The model under review builds one solid part; all positions refer to its coordinate system, in mm. A direction names the side the tool comes from. Give positions to 0.01 mm unless a question says otherwise; leave off trailing zeros. Order: outer loops, then holes, each group sorted by start corner. A loop starts at its lowest first (then second) coordinate and runs counter-clockwise, first axis right, second up. Notation, with made-up numbers: (-10, 32.25) - (45, 32.25) arc R14 cw to (45, 56.25) - close; hole circle Ø5 at (13.25, 31). An arc over 180 degrees is marked (long way). Use CSV: the item, a comma, the result in double quotes.
```python
from build123d import *
from OCP.BRepFilletAPI import BRepFilletAPI_MakeChamfer

# Parameters (mm, degrees)
SKETCH1_W           = 160
SKETCH1_H           = 4
BOSS_EXTRUDE1_DEPTH = 91
SKETCH2_W           = 5
SKETCH2_H           = 75
BOSS_EXTRUDE2_DEPTH = 91
SKETCH3_W           = 91
SKETCH3_H           = 5
BOSS_EXTRUDE3_DEPTH = 70
SKETCH4_W           = 5
SKETCH4_H           = 7
CUT_EXTRUDE1_DEPTH  = 91
SKETCH5_R           = 1.75
CUT_EXTRUDE2_DEPTH  = 91
SKETCH6_W           = 3
SKETCH6_H           = 3
CUT_EXTRUDE3_DEPTH  = 91
SKETCH7_R           = 1.65
CUT_EXTRUDE4_DEPTH  = 91
SKETCH8_W           = 20
SKETCH8_H           = 20
BOSS_EXTRUDE4_DEPTH = 6
CHAMFER1_SIZE       = 6
CHAMFER1_SIZE_2     = 4.201245229
SKETCH9_W           = 20
SKETCH9_H           = 20
BOSS_EXTRUDE5_DEPTH = 6
CHAMFER2_SIZE       = 6
CHAMFER2_SIZE_2     = 4.201245229
SKETCH10_W          = 4
SKETCH10_H          = 7
CUT_EXTRUDE5_DEPTH  = 6
SKETCH11_R          = 1.6
CUT_EXTRUDE6_DEPTH  = 6


with BuildPart() as part:
    # Sketch1 → Boss-Extrude1 (new body)
    with BuildSketch(Plane.XY):
        with Locations((80, 2)):
            Rectangle(SKETCH1_W, SKETCH1_H)
    extrude(amount=-BOSS_EXTRUDE1_DEPTH)

    # Sketch2 → Boss-Extrude2 (add)
    with BuildSketch(Plane.XY):
        with Locations((72.5, 41.5)):
            Rectangle(SKETCH2_W, SKETCH2_H)
    extrude(amount=-BOSS_EXTRUDE2_DEPTH)

    # Sketch3 → Boss-Extrude3 (add)
    with BuildSketch(Plane.ZY.offset(-70)):
        with Locations((-45.5, 76.5)):
            Rectangle(SKETCH3_W, SKETCH3_H)
    extrude(amount=BOSS_EXTRUDE3_DEPTH)

    # Sketch4 → Cut-Extrude1 (cut)
    with BuildSketch(Plane(origin=(0, 4, 0), x_dir=(1, 0, 0), z_dir=(0, 1, 0))):
        with Locations((59.5, 9.5)):
            Rectangle(SKETCH4_W, SKETCH4_H)
    extrude(amount=-CUT_EXTRUDE1_DEPTH, mode=Mode.SUBTRACT)

    # Sketch5 → Cut-Extrude2 (cut)
    with BuildSketch(Plane(origin=(0, 4, 0), x_dir=(1, 0, 0), z_dir=(0, 1, 0))):
        with Locations(Location((11, 24, 0), (0, 0, 270))):
            Circle(SKETCH5_R)
        with Locations(Location((39, 24, 0), (0, 0, 270))):
            Circle(SKETCH5_R)
        with Locations(Location((6, 76, 0), (0, 0, 270))):
            Circle(SKETCH5_R)
    extrude(amount=-CUT_EXTRUDE2_DEPTH, mode=Mode.SUBTRACT)

    # Sketch6 → Cut-Extrude3 (cut)
    with BuildSketch(Plane(origin=(0, 4, 0), x_dir=(1, 0, 0), z_dir=(0, 1, 0))):
        with Locations((36.5, 15.548738613)):
            Rectangle(SKETCH6_W, SKETCH6_H)
    extrude(amount=-CUT_EXTRUDE3_DEPTH, mode=Mode.SUBTRACT)

    # Sketch7 → Cut-Extrude4 (cut)
    with BuildSketch(Plane(origin=(0, 4, 0), x_dir=(1, 0, 0), z_dir=(0, 1, 0))):
        with Locations(Location((80, 48.5, 0), (0, 0, 270))):
            Circle(SKETCH7_R)
        with Locations(Location((80, 42.5, 0), (0, 0, 270))):
            Circle(SKETCH7_R)
    extrude(amount=-CUT_EXTRUDE4_DEPTH, mode=Mode.SUBTRACT)

    # Sketch8 → Boss-Extrude4 (add)
    with BuildSketch(Plane.XZ):
        with Locations((20, -10)):
            Rectangle(SKETCH8_W, SKETCH8_H)
    extrude(amount=BOSS_EXTRUDE4_DEPTH)

    # Chamfer1
    chamfer1_edges_1 = [part.edges().sort_by_distance(p)[0] for p in [
        (30, -6, -10),
    ]]
    chamfer1_side_1 = [part.faces().sort_by_distance(p)[0] for p in [
        (30, -5.915975095, -10),
    ]]
    chamfer1_edges_2 = [part.edges().sort_by_distance(p)[0] for p in [
        (20, -6, -20),
    ]]
    chamfer1_side_2 = [part.faces().sort_by_distance(p)[0] for p in [
        (20, -5.915975095, -20),
    ]]
    chamfer1_edges_3 = [part.edges().sort_by_distance(p)[0] for p in [
        (10, -6, -10),
    ]]
    chamfer1_side_3 = [part.faces().sort_by_distance(p)[0] for p in [
        (10, -5.915975095, -10),
    ]]
    chamfer1_edges_4 = [part.edges().sort_by_distance(p)[0] for p in [
        (20, -6, 0),
    ]]
    chamfer1_side_4 = [part.faces().sort_by_distance(p)[0] for p in [
        (20, -5.915975095, 0),
    ]]
    chamfer1 = BRepFilletAPI_MakeChamfer(part.part.solid().wrapped)
    for e in chamfer1_edges_1:
        chamfer1.Add(CHAMFER1_SIZE - 0.0001, CHAMFER1_SIZE_2 - 0.0001, e.wrapped, chamfer1_side_1[0].wrapped)
    for e in chamfer1_edges_2:
        chamfer1.Add(CHAMFER1_SIZE - 0.0001, CHAMFER1_SIZE_2 - 0.0001, e.wrapped, chamfer1_side_2[0].wrapped)
    for e in chamfer1_edges_3:
        chamfer1.Add(CHAMFER1_SIZE - 0.0001, CHAMFER1_SIZE_2 - 0.0001, e.wrapped, chamfer1_side_3[0].wrapped)
    for e in chamfer1_edges_4:
        chamfer1.Add(CHAMFER1_SIZE - 0.0001, CHAMFER1_SIZE_2 - 0.0001, e.wrapped, chamfer1_side_4[0].wrapped)
    add(Compound.cast(chamfer1.Shape()), mode=Mode.REPLACE)  # a hair under: the kernel refuses the full size

    # Sketch9 → Boss-Extrude5 (add)
    with BuildSketch(Plane.XZ):
        with Locations((20, -81)):
            Rectangle(SKETCH9_W, SKETCH9_H)
        with Locations((140, -81)):
            Rectangle(SKETCH9_W, SKETCH9_H)
        with Locations((140, -10)):
            Rectangle(SKETCH9_W, SKETCH9_H)
    extrude(amount=BOSS_EXTRUDE5_DEPTH)

    # Chamfer2
    chamfer2_edges_1 = [part.edges().sort_by_distance(p)[0] for p in [
        (30, -6, -81),
    ]]
    chamfer2_side_1 = [part.faces().sort_by_distance(p)[0] for p in [
        (30, -5.915975095, -81),
    ]]
    chamfer2_edges_2 = [part.edges().sort_by_distance(p)[0] for p in [
        (20, -6, -91),
    ]]
    chamfer2_side_2 = [part.faces().sort_by_distance(p)[0] for p in [
        (20, -5.915975095, -91),
    ]]
    chamfer2_edges_3 = [part.edges().sort_by_distance(p)[0] for p in [
        (140, -6, -91),
    ]]
    chamfer2_side_3 = [part.faces().sort_by_distance(p)[0] for p in [
        (140, -5.915975095, -91),
    ]]
    chamfer2_edges_4 = [part.edges().sort_by_distance(p)[0] for p in [
        (10, -6, -81),
    ]]
    chamfer2_side_4 = [part.faces().sort_by_distance(p)[0] for p in [
        (10, -5.915975095, -81),
    ]]
    chamfer2_edges_5 = [part.edges().sort_by_distance(p)[0] for p in [
        (20, -6, -71),
    ]]
    chamfer2_side_5 = [part.faces().sort_by_distance(p)[0] for p in [
        (20, -5.915975095, -71),
    ]]
    chamfer2_edges_6 = [part.edges().sort_by_distance(p)[0] for p in [
        (150, -6, -81),
    ]]
    chamfer2_side_6 = [part.faces().sort_by_distance(p)[0] for p in [
        (150, -5.915975095, -81),
    ]]
    chamfer2_edges_7 = [part.edges().sort_by_distance(p)[0] for p in [
        (130, -6, -81),
    ]]
    chamfer2_side_7 = [part.faces().sort_by_distance(p)[0] for p in [
        (130, -5.915975095, -81),
    ]]
    chamfer2_edges_8 = [part.edges().sort_by_distance(p)[0] for p in [
        (140, -6, -71),
    ]]
    chamfer2_side_8 = [part.faces().sort_by_distance(p)[0] for p in [
        (140, -5.915975095, -71),
    ]]
    chamfer2_edges_9 = [part.edges().sort_by_distance(p)[0] for p in [
        (130, -6, -10),
    ]]
    chamfer2_side_9 = [part.faces().sort_by_distance(p)[0] for p in [
        (130, -5.915975095, -10),
    ]]
    chamfer2_edges_10 = [part.edges().sort_by_distance(p)[0] for p in [
        (140, -6, -20),
    ]]
    chamfer2_side_10 = [part.faces().sort_by_distance(p)[0] for p in [
        (140, -5.915975095, -20),
    ]]
    chamfer2_edges_11 = [part.edges().sort_by_distance(p)[0] for p in [
        (150, -6, -10),
    ]]
    chamfer2_side_11 = [part.faces().sort_by_distance(p)[0] for p in [
        (150, -5.915975095, -10),
    ]]
    chamfer2_edges_12 = [part.edges().sort_by_distance(p)[0] for p in [
        (140, -6, 0),
    ]]
    chamfer2_side_12 = [part.faces().sort_by_distance(p)[0] for p in [
        (140, -5.915975095, 0),
    ]]
    chamfer2 = BRepFilletAPI_MakeChamfer(part.part.solid().wrapped)
    for e in chamfer2_edges_1:
        chamfer2.Add(CHAMFER2_SIZE - 0.0001, CHAMFER2_SIZE_2 - 0.0001, e.wrapped, chamfer2_side_1[0].wrapped)
    for e in chamfer2_edges_2:
        chamfer2.Add(CHAMFER2_SIZE - 0.0001, CHAMFER2_SIZE_2 - 0.0001, e.wrapped, chamfer2_side_2[0].wrapped)
    for e in chamfer2_edges_3:
        chamfer2.Add(CHAMFER2_SIZE - 0.0001, CHAMFER2_SIZE_2 - 0.0001, e.wrapped, chamfer2_side_3[0].wrapped)
    for e in chamfer2_edges_4:
        chamfer2.Add(CHAMFER2_SIZE - 0.0001, CHAMFER2_SIZE_2 - 0.0001, e.wrapped, chamfer2_side_4[0].wrapped)
    for e in chamfer2_edges_5:
        chamfer2.Add(CHAMFER2_SIZE - 0.0001, CHAMFER2_SIZE_2 - 0.0001, e.wrapped, chamfer2_side_5[0].wrapped)
    for e in chamfer2_edges_6:
        chamfer2.Add(CHAMFER2_SIZE - 0.0001, CHAMFER2_SIZE_2 - 0.0001, e.wrapped, chamfer2_side_6[0].wrapped)
    for e in chamfer2_edges_7:
        chamfer2.Add(CHAMFER2_SIZE - 0.0001, CHAMFER2_SIZE_2 - 0.0001, e.wrapped, chamfer2_side_7[0].wrapped)
    for e in chamfer2_edges_8:
        chamfer2.Add(CHAMFER2_SIZE - 0.0001, CHAMFER2_SIZE_2 - 0.0001, e.wrapped, chamfer2_side_8[0].wrapped)
    for e in chamfer2_edges_9:
        chamfer2.Add(CHAMFER2_SIZE - 0.0001, CHAMFER2_SIZE_2 - 0.0001, e.wrapped, chamfer2_side_9[0].wrapped)
    for e in chamfer2_edges_10:
        chamfer2.Add(CHAMFER2_SIZE - 0.0001, CHAMFER2_SIZE_2 - 0.0001, e.wrapped, chamfer2_side_10[0].wrapped)
    for e in chamfer2_edges_11:
        chamfer2.Add(CHAMFER2_SIZE - 0.0001, CHAMFER2_SIZE_2 - 0.0001, e.wrapped, chamfer2_side_11[0].wrapped)
    for e in chamfer2_edges_12:
        chamfer2.Add(CHAMFER2_SIZE - 0.0001, CHAMFER2_SIZE_2 - 0.0001, e.wrapped, chamfer2_side_12[0].wrapped)
    add(Compound.cast(chamfer2.Shape()), mode=Mode.REPLACE)  # a hair under: the kernel refuses the full size

    # Sketch10 → Cut-Extrude5 (cut)
    with BuildSketch(Plane(origin=(0, 4, 0), x_dir=(1, 0, 0), z_dir=(0, 1, 0))):
        with Locations((125, 45.5)):
            Rectangle(SKETCH10_W, SKETCH10_H)
    extrude(amount=-CUT_EXTRUDE5_DEPTH, mode=Mode.SUBTRACT)

    # Sketch11 → Cut-Extrude6 (cut)
    with BuildSketch(Plane.ZY.offset(-70)):
        with Locations((-70, 64.80201774)):
            Circle(SKETCH11_R)
        with Locations((-55.8, 41.80201774)):
            Circle(SKETCH11_R)
    extrude(amount=-CUT_EXTRUDE6_DEPTH, mode=Mode.SUBTRACT)


solid = part.part
```
Item 1: Clearance check with flat-ended pins moving along their axes: pin 1 (2.5 mm diameter, centred on y = 41.8, z = -55.8, fed in from +X); pin 2 (4 mm diameter, centred on y = 64.8, z = -70, fed in from +X); pin 3 (1 mm diameter, centred on x = 74, y = 35, fed in from +Z); pin 4 (10 mm diameter, centred on x = 42, z = -73.5, fed in from -Y). State where each tip first meets the part, or that it passes through.
Results list:
pin 1,"passes through"
pin 2,"stops at x = 75"
pin 3,"stops at z = 0"
pin 4,"stops at y = 0"
Item 2: Wall thickness on L1, parallel to X at y = 1, z = -24; L2, parallel to Z at x = 80, y = 1; L3, parallel to Y at x = 14, z = -63: over which ranges is each line inside the solid? List them lowest first.
Results list:
L1,"x = 0 to 9.25, 12.75 to 37.25, 40.75 to 160"
L2,"z = -91 to -50.15, -46.85 to -44.15, -40.85 to 0"
L3,"y = 0 to 4, 74 to 79"
Item 3: Mouldability with a two-part tool opening along Y and no side actions: class faces 1 (the face through (35, 4, -45)), 2 (the face through (160, 2, -45)), 3 (the face through (147.9, -3, -81.1)) as pulls with the +Y half, pulls with the -Y half, needs draft (parallel to the pull), parting line crosses it, or undercut.
Results list:
face 1,"undercut"
face 2,"needs draft"
face 3,"pulls with the -Y half"
Item 4: Take a section at A-A, the plane x = 80. Give the boundary of the cut face in (y, z).
Results list:
outline,"(0, -91) - (4, -91) - (4, -50.15) - (0, -50.15) - close; (0, -46.85) - (4, -46.85) - (4, -44.15) - (0, -44.15) - close; (0, -40.85) - (4, -40.85) - (4, 0) - (0, 0) - close"
Item 5: Tool access review of faces 4 (the face through (57, 2, -9)), 5 (the face through (70, 39, -45)), 6 (the face through (125, 2, -49)): name each direction out of +Z, -Z, +X, -X, +Y, -Y from which nothing blocks a thin tool from reaching the whole face with its end or side.
Results list:
face 4,"-Y"
face 5,"+Z, -Z, -X"
face 6,"+Y, -Y"
Item 6: Take a section at C-C, the plane z = -24. Give the boundary of the cut face in (x, y).
Results list:
outline,"(0, 0) - (9.25, 0) - (9.25, 4) - (0, 4) - close; (0, 74) - (70, 74) - (70, 4) - (40.75, 4) - (40.75, 0) - (160, 0) - (160, 4) - (75, 4) - (75, 79) - (0, 79) - close; (12.75, 0) - (37.25, 0) - (37.25, 4) - (12.75, 4) - close"
